```python
from build123d import *

# Parameters (mm, degrees)
SKETCH1_R           = 2
SKETCH1_R_2         = 1.5
BOSS_EXTRUDE1_DEPTH = 1.5
SCALE1_SCALE        = 1.5


with BuildPart() as part:
    # Sketch1 → Boss-Extrude1 (new, symmetric)
    with BuildSketch(Plane(origin=(0, 0, 0), x_dir=(1, 0, 0), z_dir=(0, 1, 0))):
        with BuildLine():
            ThreePointArc((-18.5, 4), (-22.5, 0), (-18.5, -4))
            Line((-18.5, -4), (-12.5, -4))
            ThreePointArc((-12.5, -4), (-10.036924503, -2.516685226), (-7.208497378, -2))
            Line((-7.208497378, -2), (8.627016654, -2))
            ThreePointArc((8.627016654, -2), (10.627016654, -2.254033308), (12.5, -3))
            Line((12.5, -3), (18.5, -3))
            ThreePointArc((18.5, -3), (21.5, 0), (18.5, 3))
            Line((18.5, 3), (12.5, 3))
            ThreePointArc((12.5, 3), (10.627016654, 2.254033308), (8.627016654, 2))
            Line((8.627016654, 2), (-7.208497378, 2))
            ThreePointArc((-7.208497378, 2), (-10.036924503, 2.516685226), (-12.5, 4))
            Line((-12.5, 4), (-18.5, 4))
        make_face()
        with Locations(Location((-18.5, 0, 0), (0, 0, 270))):
            Circle(SKETCH1_R, mode=Mode.SUBTRACT)
        with Locations(Location((18.5, 0, 0), (0, 0, 270))):
            Circle(SKETCH1_R_2, mode=Mode.SUBTRACT)
    extrude(amount=BOSS_EXTRUDE1_DEPTH, both=True)


with BuildPart() as part_1:
    # Scale1: scaled about (-1.682409561, 0, 0)
    add(part.part.scale(SCALE1_SCALE).moved(Location((0.841204781, 0, 0))))


solid = part_1.part
```
Design review of the part built by this model. Coordinates are the model's own, in mm. A direction names the side the tool comes from. Give positions to 0.01 mm unless a question says otherwise; leave off trailing zeros. Loops run counter-clockwise (first coordinate to the right, second up) from the corner with the lowest first, then second, coordinate; pieces in that order, holes last. Notation, with made-up numbers: M 78,12.25 L 115,12.25 A22 cw 115,34.25 Z; hole C 70,26 d8. An arc over 180 degrees is marked long. Return JSON: item names as keys, results as strings. Group by question number.
Item 1: For probe 1 along X at (y, z) = (0.8, 0); probe 2 along X at (y, z) = (-1.3, 0.25); probe 3 along Z at (x, y) = (9.5, 1.6), list the stretches that pass through material, from the lowest coordinate up.
Item 2: We need section B-B (z = 0). Give the boundary of the cut face in (x, y).
Item 3: We need section D-D (x = -12). Give the boundary of the cut face in (y, z).
Item 4: Tool access review of faces 1 (the flat face through (24, 0, 4.5)), 2 (the flat face through (2, 0, 3)), 3 (the flat face through (2, 0, -3)): name each direction out of +Z, -Z, +X, -X, +Y, -Y from which nothing blocks a thin tool from reaching the whole face with its end or side.
Item 5: We need section A-A (y = 0.8). Give the boundary of the cut face in (x, z), and give its area (3 significant figures).
Item 6: We need section C-C (x = 11). Give the boundary of the cut face in (y, z).
Item 7: Insertion check: pin 1 Ø1 at (y, z) = (-0.5, 1) entering from +X; pin 2 Ø1.3 at (x, y) = (-2, 0) entering from +Z; pin 3 Ø2 at (x, y) = (25, -0.5) entering from -Z. Each pin has a flat end and moves straight along its axis. Give the tip position at first contact, or say it passes through.
Output:
{
 "1": {"probe 1": "x = -32.91 to -29.91, -23.91 to 26.34, 30.84 to 33.09", "probe 2": "x = -32.9 to -29.9, -23.92 to 26.36, 30.83 to 33.08", "probe 3": "z = -3 to 3"},
 "2": {"outline": "M -32.91,-2.25 L -29.91,-2.25 L -29.91,2.25 L -32.91,2.25 Z; M -23.91,-2.25 L 26.34,-2.25 L 26.34,2.25 L -23.91,2.25 Z; M 30.84,-2.25 L 33.09,-2.25 L 33.09,2.25 L 30.84,2.25 Z"},
 "3": {"outline": "M -2.25,-3.17 L 2.25,-3.17 L 2.25,3.17 L -2.25,3.17 Z"},
 "4": {"face 1": "+Z, +X, +Y, -Y", "face 2": "+Z, +Y, -Y", "face 3": "-Z, +Y, -Y"},
 "5": {"outline": "M -26.91,-6 L -17.91,-6 A12 cw -9.97,-3 L 13.78,-3 A12 cw 19.59,-4.5 L 28.59,-4.5 A4.5 ccw 28.59,4.5 L 19.59,4.5 A12 cw 13.78,3 L -9.97,3 A12 cw -17.91,6 L -26.91,6 A6 ccw Z; hole C -26.91,0 d6; hole C 28.59,0 d4.5", "area": "479 mm^2"},
 "6": {"outline": "M -2.25,-3 L 2.25,-3 L 2.25,3 L -2.25,3 Z"},
 "7": {"pin 1": "stops at x = 33.06", "pin 2": "stops at z = 3", "pin 3": "stops at z = -4.5"}
}
